Geometry: final body of the model. Coordinates: model frame, mm. Face numbers are marked on the shaded views. Round coordinates to 2 decimals unless told otherwise and drop trailing zeros. Order: outer loops, then holes, each group sorted by start corner. A loop starts at its lowest first (then second) coordinate and runs counter-clockwise, first axis right, second up. Notation, with made-up numbers: (30.5, -3.75) - (66.5, -3.75) arc R9 cw to (66.5, 8.25) - close; hole circle Ø8 at (0.5, 85). An arc over 180 degrees is marked (long way). Put each result on its own line as item: value. Start each with the question number.
(1) Section D-D (z = -11.5). Output: boundary loops of the cut face in (x, y).
(2) Pin query (flat end, axial travel): P1, Ø4, axis at y = -5, z = -7.5, coming from the +X side. Return the tip coordinate at first contact, or that it passes through.
(3) Section A-A (y = -5.75). Output: boundary loops of the cut face in (x, z), and give its area (3 significant figures).
(4) Pull-direction query (X, two-part tool) for the marked faces 1, 2 and 3; classes: released by +X, released by -X, zero draft, split by the parting line, or undercut.
(5) Section C-C (x = 5). Output: boundary loops of the cut face in (y, z), and give its area (3 significant figures).
(6) Section B-B (z = -6). Output: boundary loops of the cut face in (x, y).
(7) Material intervals for L1, parallel to Y at x = -5, z = -7.5; L2, parallel to X at y = -5, z = -3.5; L3, parallel to Z at x = 9.5, y = -5, sorted ascending. Write a range as [from, to].
from build123d import *

# Parameters (mm, degrees)
SCHIZZO1_W                   = 31.958658916
SCHIZZO1_H                   = 15
ESTRUSIONE_ESTRUSIONE1_DEPTH = 10
SCHIZZO4_R                   = 2.5
TAGLIO_ESTRUSIONE1_DEPTH     = 25.103941586
SCHIZZO5_R                   = 2.5
TAGLIO_ESTRUSIONE2_DEPTH     = 37.692722435


with BuildPart() as part:
    # Schizzo1 → Estrusione-Estrusione1 (new body)
    with BuildSketch(Plane(origin=(0, 0, 0), x_dir=(1, 0, 0), z_dir=(0, 1, 0))):
        with Locations((-0.020670542, 7.5)):
            Rectangle(SCHIZZO1_W, SCHIZZO1_H)
    extrude(amount=-ESTRUSIONE_ESTRUSIONE1_DEPTH)

    # Schizzo4 → Taglio-Estrusione1 (cut, through all)
    with BuildSketch(Plane.XY):
        with Locations((-0.020670542, -5)):
            Circle(SCHIZZO4_R)
    extrude(amount=-TAGLIO_ESTRUSIONE1_DEPTH, mode=Mode.SUBTRACT)

    # Schizzo5 → Taglio-Estrusione2 (cut, through all)
    with BuildSketch(Plane(origin=(15.958658916, 0, 0), x_dir=(0, 0, -1), z_dir=(1, 0, 0))):
        with Locations((7.5, -5)):
            Circle(SCHIZZO5_R)
    extrude(amount=-TAGLIO_ESTRUSIONE2_DEPTH, mode=Mode.SUBTRACT)


solid = part.part
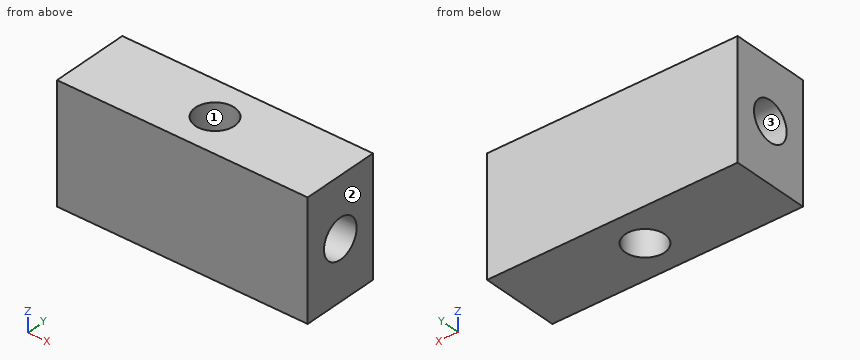
Checks:
1. outline: (-16, -10) - (15.96, -10) - (15.96, 0) - (-16, 0) - close; hole circle Ø5 at (-0.02, -5)
2. P1: passes through
3. outline: (-16, -15) - (-2.41, -15) - (-2.41, -9.88) - (-16, -9.88) - close; (-16, -5.12) - (-2.41, -5.12) - (-2.41, 0) - (-16, 0) - close; (2.36, -15) - (15.96, -15) - (15.96, -9.88) - (2.36, -9.88) - close; (2.36, -5.12) - (15.96, -5.12) - (15.96, 0) - (2.36, 0) - close
3. area: 278 mm²
4. face 1: undercut
4. face 2: released by +X
4. face 3: zero draft
5. outline: (-10, -15) - (0, -15) - (0, 0) - (-10, 0) - close; hole circle Ø5 at (-5, -7.5)
5. area: 130 mm²
6. outline: (-16, -10) - (15.96, -10) - (15.96, -7) - (1.48, -7) arc R2.5 cw to (-1.52, -7) - (-16, -7) - close; (-16, -3) - (-1.52, -3) arc R2.5 cw to (1.48, -3) - (15.96, -3) - (15.96, 0) - (-16, 0) - close
7. L1: y = [-10, -7.5], [-2.5, 0]
7. L2: x = [-16, -2.52], [2.48, 15.96]
7. L3: z = [-15, -10], [-5, 0]
